```python
from build123d import *


with BuildPart() as part:
    # Sketch1 → Revolve1 (revolve)
    with BuildSketch(Plane(origin=(0, 0, 0), x_dir=(0, 0, -1), z_dir=(1, 0, 0))):
        with BuildLine():
            Line((1.75, 9), (1.75, 10))
            Line((1.75, 10), (7, 10))
            Line((7, 10), (7, 8))
            Line((7, 8), (6, 8))
            Line((6, 8), (6, 0))
            Line((6, 0), (0, 0))
            Line((0, 0), (0, 9.5))
            ThreePointArc((0, 9.5), (0.910013736, 9.372548077), (1.75, 9))
        make_face()
    revolve(axis=Axis((0, 0, 0), (0, 1, 0)))


solid = part.part
```
Check sheet for the modelled part. Datum: model origin and axes. Units: mm. A direction names the side the tool comes from. Coordinates: 2 decimals unless noted, no trailing zeros. Loops run counter-clockwise (first coordinate to the right, second up) from the corner with the lowest first, then second, coordinate; pieces in that order, holes last. Notation, with made-up numbers: M 66,69.5 L 83,69.5 A17 cw 83,90.5 Z; hole C -22,-18 d5. An arc over 180 degrees is marked long. Answer as a JSON object with one key per item and string values.
1. Release check for a two-part mould opening along X. For faces 3 (the flat face through (0, 0, 0)), 4 (the cylindrical face through (0.67, 9.507, -1.617)), 5 (the cylindrical face through (2.681, 8.986, -6.466)) record: pulls with the +X half, pulls with the -X half, needs draft (parallel to the pull), parting line crosses it, or undercut.
Outcome:
{"face 3": "needs draft", "face 4": "undercut", "face 5": "parting line crosses it"}
2. Depth check by flat-ended pin: P1, Ø6, axis at y = 1, z = 1.5, coming from the -X side; P2, Ø1, axis at x = -2.5, y = 3, coming from the -Z side; P3, Ø5, axis at y = 3, z = 2, coming from the +X side; P4, Ø5.5, axis at x = 0, z = 0, coming from the -Y side. Enter the tip coordinate at first touch or a pass-through.
Outcome:
{"P1": "x = -6", "P2": "z = -5.66", "P3": "x = 6", "P4": "y = 0"}
3. Access from +Z, -Z, +X, -X, +Y, -Y to the whole of each face (thin tool, end or side, straight path). Record for faces 1 (the flat face through (1.5, 10, 1.5)), 2 (the flat face through (-2, 8, -6)).
Outcome:
{"face 1": "+Z, -Z, +X, -X, +Y", "face 2": "-Y"}
4. Sectioned sample at D-D on x = -4.75. Record the cut outline in (y, z), and give its area (3 significant figures).
Outcome:
{"outline": "M 0,-3.67 L 8,-3.67 L 8,-5.14 L 10,-5.14 L 10,5.14 L 8,5.14 L 8,3.67 L 0,3.67 Z", "area": "79.2 mm²"}
5. Sectioned sample at B-B on z = 5.25. Record the cut outline in (x, y), and give its area (3 significant figures).
Outcome:
{"outline": "M -4.63,8 L -2.9,8 L -2.9,0 L 2.9,0 L 2.9,8 L 4.63,8 L 4.63,10 L -4.63,10 Z", "area": "65.0 mm²"}
6. Sectioned sample at C-C on y = 3. Record the cut outline in (x, z).
Outcome:
{"outline": "C 0,0 d12"}
7. Scan lines: L1, parallel to Z at x = 0, y = 9.85; L2, parallel to Y at x = -1.5, z = 6; L3, parallel to Y at x = 0.5, z = -1. Record each from-to range of solid material in increasing order. Write a range as from..to.
Outcome:
{"L1": "-7..-1.75, 1.75..7", "L2": "8..10", "L3": "0..9.31"}
